Job drawing, mm, ordinate dimensions from the low corner. One solid piece. Give positions to 0.01 mm unless a question says otherwise; leave off trailing zeros. Order: outer loops, then holes, each group sorted by start corner. A loop starts at its lowest first (then second) coordinate and runs counter-clockwise, first axis right, second up. Notation, with made-up numbers: M 47,80.5 L 78,80.5 A12 ccw 78,103.5 Z; hole C -2,6.5 d2. An arc over 180 degrees is marked long. Put each result on its own line as item: value. Start each with the question number.
1) Cut at A-A (y = 181.5). Write the cut outline in (x, z), and give its area (3 significant figures).
2) Cut at B-B (z = 21). Write the cut outline in (x, y).
3) Pin check, flat tips, straight feed: pin 1 (4 mm diameter, centred on y = 533, z = 65, fed in from +X); pin 2 (1.5 mm diameter, centred on x = 594.5, z = 29, fed in from +Y). Stop position of each tip, or through.
4) Drill centre line: line 1 (Y direction, x = 1377, z = 35.5). Where is it in solid material? Low to high. Write a range as [from, to].
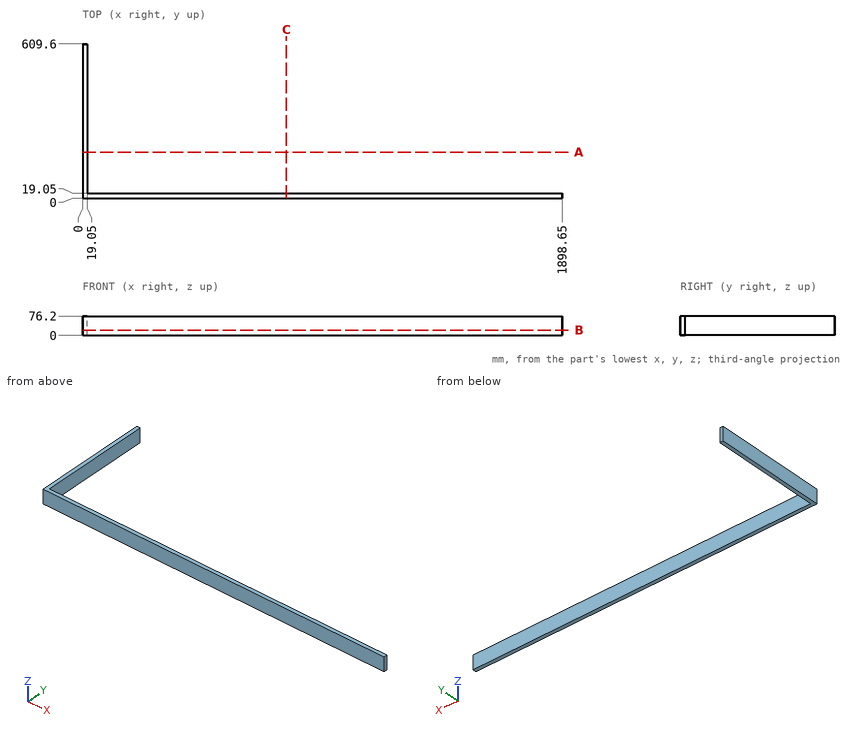
Solution:
1. outline: M 0,0 L 19.05,0 L 19.05,76.2 L 0,76.2 Z
1. area: 1,450 mm²
2. outline: M 0,0 L 1898.65,0 L 1898.65,19.05 L 19.05,19.05 L 19.05,609.6 L 0,609.6 Z
3. pin 1: x = 19.05
3. pin 2: y = 19.05
4. line 1: [0, 19.05]
